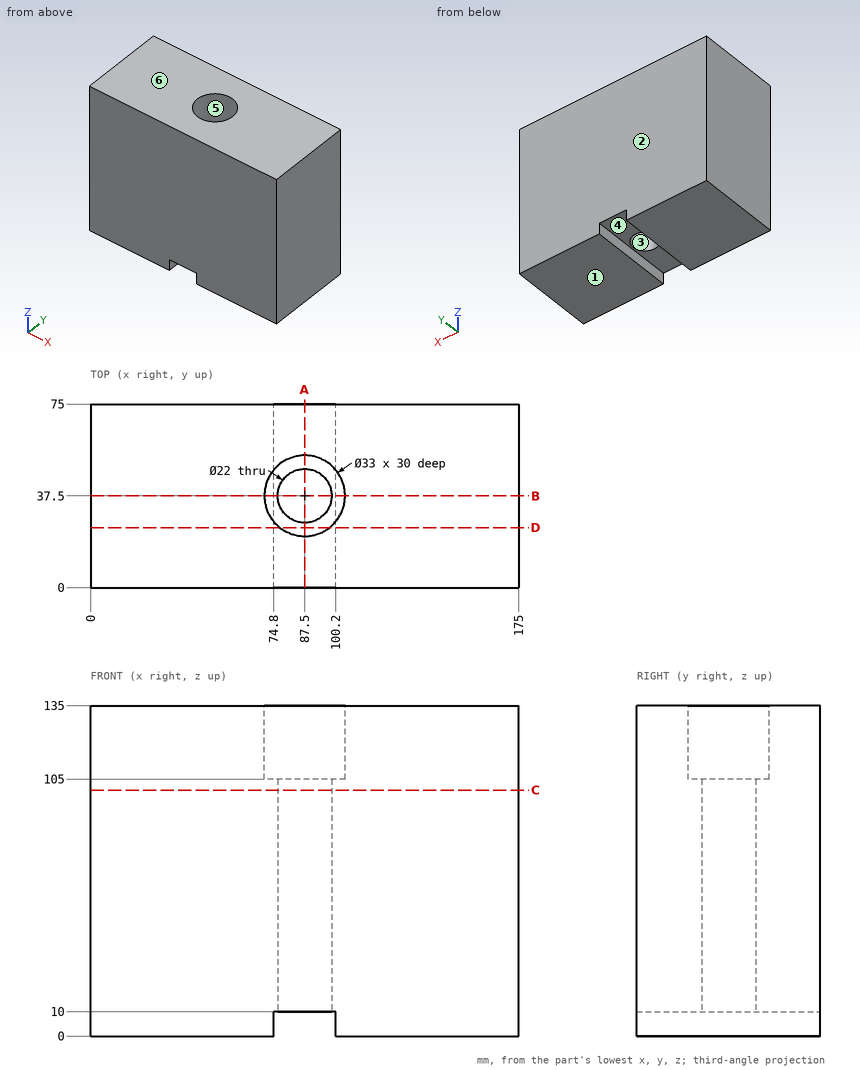
Could you check a few things on this drawing? It's one solid part, dimensions in mm from its lowest x, y, z. A direction names the side the tool comes from. Round coordinates to 2 decimals unless told otherwise and drop trailing zeros. Order: outer loops, then holes, each group sorted by start corner. A loop starts at its lowest first (then second) coordinate and runs counter-clockwise, first axis right, second up. Notation, with made-up numbers: M -17.75,23.25 L 5.25,23.25 A35 cw 5.25,57.25 Z; hole C -27.5,67 d7. An arc over 180 degrees is marked long. One line per question, with ' | ' between items. Start each with the question number.
(1) For the marked faces 4, 5 and 6, which set-ups out of +Z, -Z, +X, -X, +Y, -Y let a thin tool reach every point of the face, with its end or its side?
(2) Suppose I cut it at C-C on z = 100.5. List the corners of the cut face in (x, y) for me, then the cut area to 3 significant figures.
(3) For P1, Ø12, axis at x = 85, y = 32, coming from the +Z side; P2, Ø12.5, axis at x = 88.5, y = 35.5, coming from the -Z side, each with a flat end and sliding along its axis, tell me the tip position at first contact or that it passes through.
(4) Thinking about a two-plate mould opening in Y: for the marked faces 1, 2 and 3, which applies, +Y half, -Y half, draft (parallel to the pull), parting line (faces both ways), or undercut?
(5) Suppose I cut it at B-B on y = 37.5. List the corners of the cut face in (x, z) for me.
(6) Please list where these lines run through material, in increasing order: line 1 along Y through (x, z) = (87.5, 81); line 2 along X through (y, z) = (37, 45); line 3 along X through (y, z) = (37, 112).
(7) Suppose I cut it at D-D on y = 24.5. List the corners of the cut face in (x, z) for me, then the cut area to 3 significant figures.
(8) Suppose I cut it at A-A on x = 87.5. List the corners of the cut face in (y, z) for me.
Geometry results:
1) face 4: -Z, +Y, -Y | face 5: +Z | face 6: +Z, +X, -X, +Y, -Y
2) outline: M 0,0 L 175,0 L 175,75 L 0,75 Z; hole C 87.5,37.5 d22 | area: 12,700 mm²
3) P1: z = 105 | P2: through
4) face 1: draft | face 2: +Y half | face 3: undercut
5) outline: M 0,0 L 74.8,0 L 74.8,10 L 76.5,10 L 76.5,105 L 71,105 L 71,135 L 0,135 Z; M 98.5,10 L 100.2,10 L 100.2,0 L 175,0 L 175,135 L 104,135 L 104,105 L 98.5,105 Z
6) line 1: 0 to 26.5, 48.5 to 75 | line 2: 0 to 76.51, 98.49 to 175 | line 3: 0 to 71.01, 103.99 to 175
7) outline: M 0,0 L 74.8,0 L 74.8,10 L 100.2,10 L 100.2,0 L 175,0 L 175,135 L 97.66,135 L 97.66,105 L 77.34,105 L 77.34,135 L 0,135 Z | area: 22,800 mm²
8) outline: M 0,10 L 26.5,10 L 26.5,105 L 21,105 L 21,135 L 0,135 Z; M 48.5,10 L 75,10 L 75,135 L 54,135 L 54,105 L 48.5,105 Z
